Build history of the part. All positions in model axes, mm. Face numbers are marked on the shaded views. A direction names the side the tool comes from. Give positions to 0.01 mm unless a question says otherwise; leave off trailing zeros. Write each loop counter-clockwise with the first axis right and the second up, starting at its lowest first coordinate (ties: lowest second). Pieces come first, ordered by that corner, then holes. Notation, with made-up numbers: (-11, 8) - (8, 8) arc R8 cw to (8, 21) - close; hole circle Ø2 at (60.25, 21.5). An arc over 180 degrees is marked (long way). Use one line per item in the form item = value. Start each with the question number.
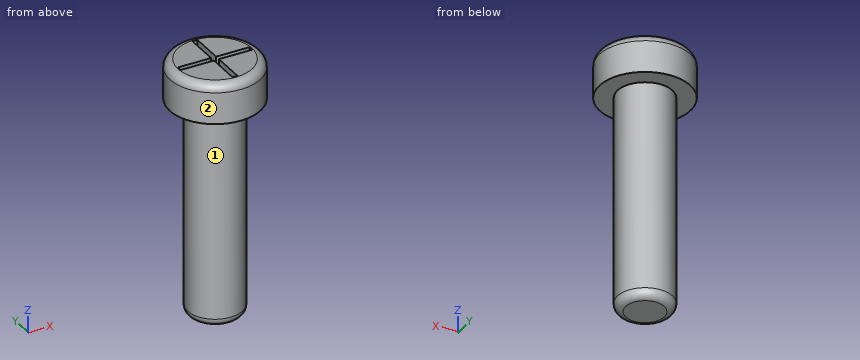
from build123d import *

# Parameters (mm, degrees)
SKICA1_R                 = 2.725
P_IDAT_VYSUNUT_M1_DEPTH  = 2.4
SKICA2_R                 = 1.65
P_IDAT_VYSUNUT_M3_DEPTH  = 13
ODEBRAT_VYSUNUT_M1_DEPTH = 1
ZAOBLIT1_R               = 0.5


with BuildPart() as part:
    # Skica1 → Přidat vysunutím1 (new body)
    with BuildSketch(Plane.XY):
        Circle(SKICA1_R)
    extrude(amount=P_IDAT_VYSUNUT_M1_DEPTH)

    # Skica2 → Přidat vysunutím3 (add)
    with BuildSketch(Plane(origin=(0, 0, 0), x_dir=(-1, 0, 0), z_dir=(0, 0, -1))):
        Circle(SKICA2_R)
    extrude(amount=P_IDAT_VYSUNUT_M3_DEPTH)

    # Skica4 → Odebrat vysunutím1 (cut)
    with BuildSketch(Plane.XY.offset(2.4)):
        Polygon((-0.15, 0.15), (-0.15, 2.15), (0.15, 2.15), (0.15, 0.15), (2.15, 0.15), (2.15, -0.15), (0.15, -0.15), (0.15, -2.15), (-0.15, -2.15), (-0.15, -0.15), (-2.15, -0.15), (-2.15, 0.15), align=None)
    extrude(amount=-ODEBRAT_VYSUNUT_M1_DEPTH, mode=Mode.SUBTRACT)

    # Zaoblit1
    zaoblit1_edges = [part.edges().sort_by_distance(p)[0] for p in [
        (-2.725, 0, 2.4),
        (1.65, 0, -13),
    ]]
    fillet(zaoblit1_edges, radius=ZAOBLIT1_R)


solid = part.part
(1) Pin check, flat tips, straight feed: pin 1 Ø0.5 at (x, z) = (-0.5, 2) entering from -Y; pin 2 Ø0.8 at (x, z) = (1.5, 2) entering from -Y; pin 3 Ø0.8 at (y, z) = (1, 2) entering from +X. Stop position of each tip, or through.
(2) Which spindle directions (+Z, -Z, +X, -X, +Y, -Y) get a long thin tool onto all of the face, cutting with end or side? Do the marked faces 1 and 2. Say none if no direction does.
(3) Wall check: line 1 (X direction, y = 0.1, z = 1.75); line 2 (Y direction, x = -0.1, z = -4.5); line 3 (Z direction, x = 1.65, y = 0.8). Give the ranges that are in metal, low to high. Write a range as from..to.
(4) Cut at C-C, the plane z = -12. Give the cut face in (x, y).
(5) Cut at A-A, the plane y = 0. Give the cut face in (x, z) (3 decimals), then the cut area to 3 significant figures.
Solution:
q1.pin_1 = -2.71
q1.pin_2 = -2.49
q1.pin_3 = 2.66
q2.face_1 = -Z
q2.face_2 = +Z, -Z
q3.line_1 = -2.72..-2.15, 2.15..2.72
q3.line_2 = -1.65..1.65
q3.line_3 = 0..2.4
q4.outline = circle Ø3.3 at (0, 0)
q5.outline = (-2.725, 0) - (-1.65, 0) - (-1.65, -12.5) arc R0.5 ccw to (-1.15, -13) - (1.15, -13) arc R0.5 ccw to (1.65, -12.5) - (1.65, 0) - (2.725, 0) - (2.725, 1.9) arc R0.5 ccw to (2.225, 2.4) - (2.15, 2.4) - (2.15, 1.4) - (-2.15, 1.4) - (-2.15, 2.4) - (-2.225, 2.4) arc R0.5 ccw to (-2.725, 1.9) - close
q5.area = 51.5 mm2
